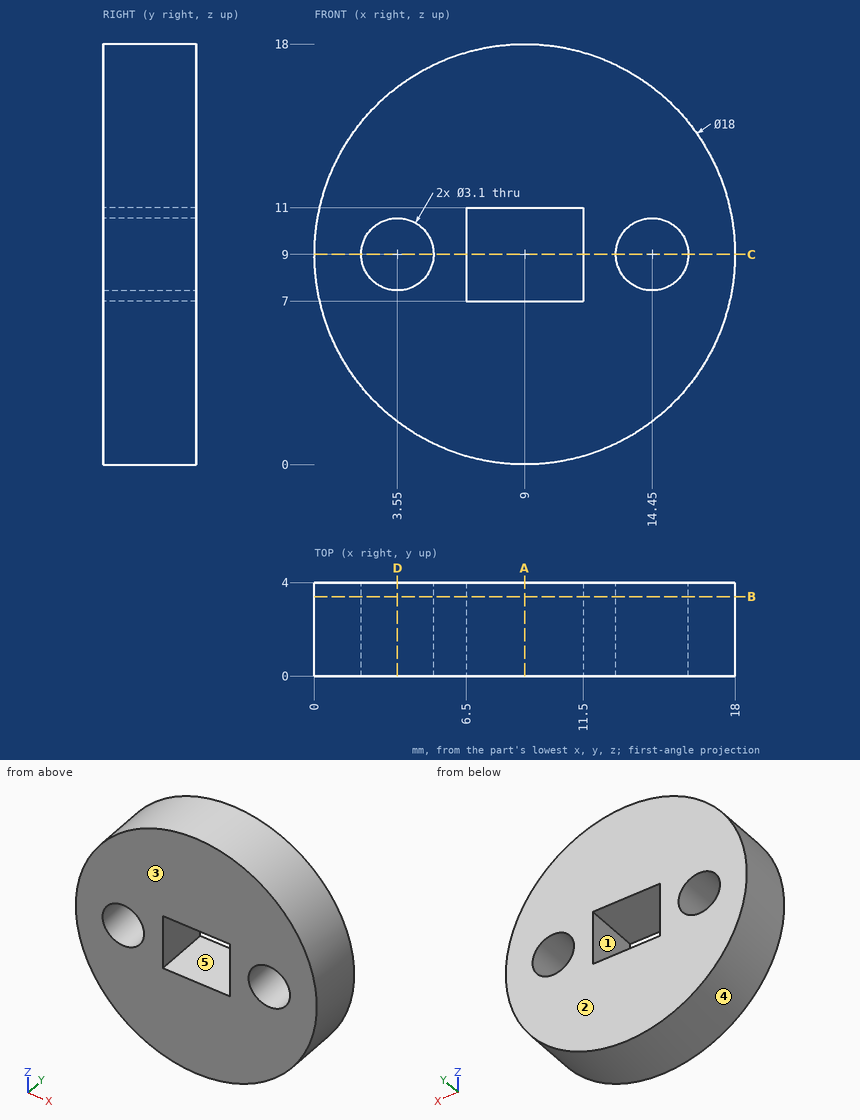
The drawing under review shows one solid part. Ordinate dimensions are in mm from its lowest x, y, z. A direction names the side the tool comes from. Give positions to 0.01 mm unless a question says otherwise; leave off trailing zeros. Write each loop counter-clockwise with the first axis right and the second up, starting at its lowest first coordinate (ties: lowest second). Pieces come first, ordered by that corner, then holes. Notation, with made-up numbers: (19, 11.5) - (78, 11.5) arc R34 ccw to (78, 46.5) - close; hole circle Ø7 at (53, 47.25). An arc over 180 degrees is marked (long way). Answer in a Markdown table with one row per item. Add a question column.
1. We need section A-A on x = 9. Write out the cut boundary in (y, z).
2. Insertion check: P1, Ø2.5, axis at x = 3.55, z = 9, coming from the +Y side; P2, Ø2, axis at y = 0.5, z = 3.5, coming from the -X side; P3, Ø2, axis at y = 3, z = 12.5, coming from the +X side; P4, Ø1.5, axis at x = 13.5, y = 2, coming from the -Z side. Each pin has a flat end and moves straight along its axis. Give the tip position at first contact, or say it passes through.
3. We need section B-B on y = 3.4. Write out the cut boundary in (x, z).
4. Tool access review of the marked faces 1 and 2: name each direction out of +Z, -Z, +X, -X, +Y, -Y from which nothing blocks a thin tool from reaching the whole face with its end or side.
5. Draft analysis for pull direction X (two halves, no side actions). For the marked faces 3, 4 and 5, state which applies: +X half, -X half, draft (parallel to the pull), parting line (faces both ways), or undercut.
6. We need section D-D on x = 3.55. Write out the cut boundary in (y, z).
7. Wall thickness on line 1 along X through (y, z) = (3.1, 9); line 2 along Z through (x, y) = (4.25, 2.55); line 3 along Z through (x, y) = (4.5, 2.1): over which ranges is each line inside the solid? List them lowest first. Write a range as [from, to].
8. We need section C-C on z = 9. Write out the cut boundary in (x, y), then the cut area to 3 significant figures.
Ans:
| question | item | result |
|---|---|---|
| 1 | outline | (0, 0) - (4, 0) - (4, 7) - (0, 7) - close; (0, 11) - (4, 11) - (4, 18) - (0, 18) - close |
| 2 | P1 | passes through |
| 2 | P2 | stops at x = 1.21 |
| 2 | P3 | stops at x = 17.65 |
| 2 | P4 | stops at z = 0.82 |
| 3 | outline | circle Ø18 at (9, 9); hole circle Ø3.1 at (3.55, 9); hole (6.5, 7) - (11.5, 7) - (11.5, 11) - (6.5, 11) - close; hole circle Ø3.1 at (14.45, 9) |
| 4 | face 1 | +Y, -Y |
| 4 | face 2 | +Z, -Z, +X, -X, +Y |
| 5 | face 3 | draft |
| 5 | face 4 | parting line |
| 5 | face 5 | undercut |
| 6 | outline | (0, 1.84) - (4, 1.84) - (4, 7.45) - (0, 7.45) - close; (0, 10.55) - (4, 10.55) - (4, 16.16) - (0, 16.16) - close |
| 7 | line 1 | x = [0, 2], [5.1, 6.5], [11.5, 12.9], [16, 18] |
| 7 | line 2 | z = [1.36, 7.62], [10.38, 16.64] |
| 7 | line 3 | z = [1.21, 7.78], [10.22, 16.79] |
| 8 | outline | (0, 0) - (2, 0) - (2, 4) - (0, 4) - close; (5.1, 0) - (6.5, 0) - (6.5, 4) - (5.1, 4) - close; (11.5, 0) - (12.9, 0) - (12.9, 4) - (11.5, 4) - close; (16, 0) - (18, 0) - (18, 4) - (16, 4) - close |
| 8 | area | 27.2 mm^2 |
